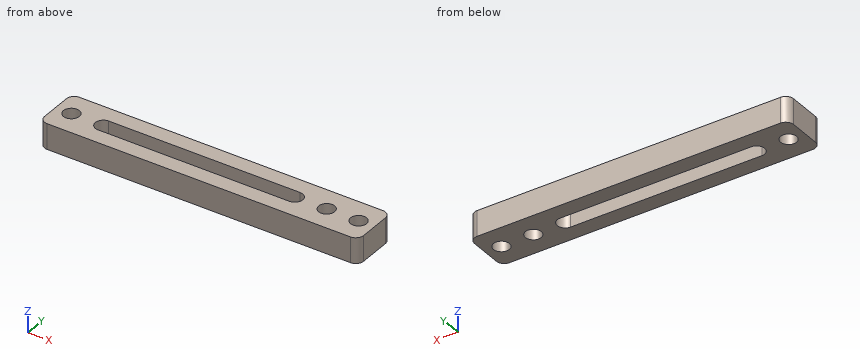
```python
from build123d import *

# Parameters (mm, degrees)
SKETCH_1_W          = 100
SKETCH_1_H          = 15
EXTRUDE_1_DEPTH     = 8
SKETCH_2_R          = 2.5
CUT_EXTRUDE_2_DEPTH = 8
FILLET_2_R          = 2.5


with BuildPart() as part:
    # Эскиз1 → Вытянуть1 (new body)
    with BuildSketch(Plane.XY):
        with Locations((50, 7.5)):
            Rectangle(SKETCH_1_W, SKETCH_1_H)
    extrude(amount=EXTRUDE_1_DEPTH)

    # Эскиз2 → Вытянуть2 (cut)
    with BuildSketch(Plane.XY.offset(8)):
        with Locations((5, 7.5)):
            Circle(SKETCH_2_R)
        with Locations((95, 7.5)):
            Circle(SKETCH_2_R)
        with Locations((85, 7.5)):
            Circle(SKETCH_2_R)
        with BuildLine():
            Line((15, 10), (75, 10))
            ThreePointArc((75, 10), (77.5, 7.5), (75, 5))
            Line((75, 5), (15, 5))
            ThreePointArc((15, 5), (12.5, 7.5), (15, 10))
        make_face()
    extrude(amount=-CUT_EXTRUDE_2_DEPTH, mode=Mode.SUBTRACT)

    # Скругление2
    fillet_2_edges = [part.edges().sort_by_distance(p)[0] for p in [
        (0, 15, 4),
        (100, 15, 4),
        (100, 0, 4),
        (0, 0, 4),
    ]]
    fillet(fillet_2_edges, radius=FILLET_2_R)


solid = part.part
```
Model file for the job. Use its own axes, mm. Coordinates: 2 decimals unless noted, no trailing zeros. Write each loop counter-clockwise with the first axis right and the second up, starting at its lowest first coordinate (ties: lowest second). Pieces come first, ordered by that corner, then holes. Notation, with made-up numbers: (52, 10) - (60, 10) arc R8 ccw to (60, 14) - close; hole circle Ø6 at (-7, 51.25). An arc over 180 degrees is marked (long way). One line per item, written item: value. Start each with the question number.
1. Flat gauge pin, fed straight in: pin 1 (4 mm diameter, centred on x = 85, y = 7.5, fed in from +Z). Where does the tip first touch, or does it go through?
2. Slice it at A-A (z = 4). Write the cut outline in (x, y), plus the area to 3 significant figures.
3. Probe line 1 (Y direction, x = 35.5, z = 6.25); line 2 (X direction, y = 7, z = 2); line 3 (Y direction, x = 94.5, z = 0.5). List the from-to ranges inside material, lowest first. Write a range as from..to.
4. Slice it at B-B (x = 24.5). Write the cut outline in (y, z).
Answers below:
1. pin 1: passes through
2. outline: (0, 2.5) arc R2.5 ccw to (2.5, 0) - (97.5, 0) arc R2.5 ccw to (100, 2.5) - (100, 12.5) arc R2.5 ccw to (97.5, 15) - (2.5, 15) arc R2.5 ccw to (0, 12.5) - close; hole circle Ø5 at (5, 7.5); hole (15, 5) - (75, 5) arc R2.5 ccw to (75, 10) - (15, 10) arc R2.5 ccw to start; hole circle Ø5 at (85, 7.5); hole circle Ø5 at (95, 7.5)
2. area: 1,120 mm^2
3. line 1: y = 0..5, 10..15
3. line 2: x = 0..2.55, 7.45..12.55, 77.45..82.55, 87.45..92.55, 97.45..100
3. line 3: y = 0..5.05, 9.95..15
4. outline: (0, 0) - (5, 0) - (5, 8) - (0, 8) - close; (10, 0) - (15, 0) - (15, 8) - (10, 8) - close
